from build123d import *

# Parameters (mm, degrees)
F0_W     = 74.2121748626
F0_H     = 53.3399991691
F1_DEPTH = 25.4
F2_R     = 5.08
F3_R     = 13.6810571513
F4_DEPTH = 31.75


with BuildPart() as f1:
    # F0 (on Top) → F1 (new body)
    with BuildSketch(Plane.XY):
        with Locations((3.6443490535, 1.9878260791)):
            Rectangle(F0_W, F0_H)
        Polygon((40.7504364848, 44.229131192), (40.7504364848, 28.6578256637), (40.7504364848, -24.6821735054), (69.5739164948, -24.6821735054), (69.5739164948, 44.229131192), align=None)
    extrude(amount=F1_DEPTH)

    # F2
    f2_edges = [f1.edges().sort_by_distance(p)[0] for p in [
        (-33.461738, 1.987826, 25.4),
        (3.644349, 28.657826, 25.4),
        (55.162176, 44.229131, 25.4),
        (18.056089, -24.682174, 25.4),
        (69.573916, 9.773479, 25.4),
    ]]
    fillet(f2_edges, radius=F2_R)

    # F3 (on face) → F4 (join)
    with BuildSketch(Plane.XY.offset(25.4)):
        Polygon((64.4939164948, 39.149131192), (40.7504364848, 39.149131192), (40.7504364848, 28.6578256637), (40.7504364848, 23.5778256637), (-28.3817383778, 23.5778256637), (-28.3817383778, -19.6021735054), (64.4939164948, -19.6021735054), align=None)
        with Locations((20.3587319702, 0)):
            Circle(F3_R, mode=Mode.SUBTRACT)
        with Locations((20.3587319702, 0)):
            Circle(F3_R)
    extrude(amount=-F4_DEPTH)


solid = f1.part
The model under review builds one solid part; all positions refer to its coordinate system, in mm. A direction names the side the tool comes from. Round coordinates to 2 decimals unless told otherwise and drop trailing zeros. Order: outer loops, then holes, each group sorted by start corner. A loop starts at its lowest first (then second) coordinate and runs counter-clockwise, first axis right, second up. Notation, with made-up numbers: (12, 26.5) -> (58, 26.5) arc R25 cw to (58, 49.5) -> close; hole circle Ø2 at (4, -12.75). An arc over 180 degrees is marked (long way). Return JSON: item names as keys, results as strings.
1. For faces 1 (the face through (53, 39.149, -3)), 2 (the face through (-28.382, 2, -3)), 3 (the face through (64.494, 9, -3)), list the 3-axis set-ups (+Z, -Z, +X, -X, +Y, -Y) from which the entire face can be reached by the end or side of a thin tool; tool diameter is ignored.
Answer block:
{"face 1": "-Z, +X, -X, +Y", "face 2": "-Z, -X, +Y, -Y", "face 3": "-Z, +X, +Y, -Y"}
2. Take a section at D-D (y = 20). Write out the cut boundary in (x, z), then the cut area to 3 significant figures.
Answer block:
{"outline": "(-33.46, 0) -> (-28.38, 0) -> (-28.38, -6.35) -> (64.49, -6.35) -> (64.49, 0) -> (69.57, 0) -> (69.57, 20.32) arc R5.08 ccw to (64.49, 25.4) -> (-28.38, 25.4) arc R5.08 ccw to (-33.46, 20.32) -> close", "area": "3,200 mm²"}
3. For L1, parallel to Y at x = 20, z = 2.5; L2, parallel to X at y = 34, z = 13.5; L3, parallel to X at y = -16, z = -3, list the stretches that pass through material, from the lowest coordinate up. Write a range as [from, to].
Answer block:
{"L1": "y = [-24.68, 28.66]", "L2": "x = [40.75, 69.57]", "L3": "x = [-28.38, 64.49]"}
4. Take a section at B-B (x = 59.5). Write out the cut boundary in (y, z).
Answer block:
{"outline": "(-24.68, 0) -> (-19.6, 0) -> (-19.6, -6.35) -> (39.15, -6.35) -> (39.15, 0) -> (44.23, 0) -> (44.23, 20.32) arc R5.08 ccw to (39.15, 25.4) -> (-19.6, 25.4) arc R5.08 ccw to (-24.68, 20.32) -> close"}
5. Insertion check: P1, Ø3, axis at x = 49, z = -4.5, coming from the +Y side; P2, Ø1.5, axis at x = -2.5, z = 0.5, coming from the +Y side; P3, Ø3, axis at x = -2.5, z = -2.5, coming from the -Y side. Each pin has a flat end and moves straight along its axis. Give the tip position at first contact, or say it passes through.
Answer block:
{"P1": "stops at y = 39.15", "P2": "stops at y = 28.66", "P3": "stops at y = -19.6"}
6. Take a section at A-A (y = 36.5). Write out the cut boundary in (x, z).
Answer block:
{"outline": "(40.75, -6.35) -> (64.49, -6.35) -> (64.49, 0) -> (69.57, 0) -> (69.57, 20.32) arc R5.08 ccw to (64.49, 25.4) -> (40.75, 25.4) -> close"}
7. Take a section at C-C (z = 13.5). Write out the cut boundary in (x, y).
Answer block:
{"outline": "(-33.46, -24.68) -> (69.57, -24.68) -> (69.57, 44.23) -> (40.75, 44.23) -> (40.75, 28.66) -> (-33.46, 28.66) -> close"}
